Read the model definition and answer for the solid it produces. Units are mm, in the model's axes. Coordinates: 2 decimals unless noted, no trailing zeros. One line per item, written item: value. Start each with the question number.
1. Consider probe 1 along X at (y, z) = (-122.5, 5.25); probe 2 along X at (y, z) = (-123, 6.75); probe 3 along Z at (x, y) = (64.5, -119.5). Determine where each line is inside the solid, lowest interval first.
2. Determine the mould class of faces 1 (the face through (-4, -105, 3.463)), 2 (the face through (-4, -98, 16)), 3 (the face through (-1.85, -108.142, 8.112)) for opening direction Y: +Y half, -Y half, draft (parallel to the pull), parting line (faces both ways), or undercut.
3. Flat-ended cylindrical pins translate along their axes: pin 1 (2 mm diameter, centred on x = -36.5, z = 5.5, fed in from -Y); pin 2 (3 mm diameter, centred on x = -8, z = 5, fed in from -Y). Find the tip coordinate at first contact, or state that the pin passes through.
```python
from build123d import *

# Parameters (mm, degrees)
SKETCH1_W           = 169.5
SKETCH1_H           = 47.45
BOSS_EXTRUDE1_DEPTH = 32
SKETCH7_R           = 154
CUT_EXTRUDE5_DEPTH  = 32
SKETCH14_W          = 169.5
SKETCH14_H          = 16
BOSS_EXTRUDE2_DEPTH = 10


with BuildPart() as part:
    # Sketch1 → Boss-Extrude1 (new body)
    with BuildSketch(Plane.XY):
        with Locations((-3.10671108, -121.862113139)):
            Rectangle(SKETCH1_W, SKETCH1_H)
    extrude(amount=BOSS_EXTRUDE1_DEPTH)

    # Sketch7 → Cut-Extrude5 (cut)
    with BuildSketch(Plane.XY.offset(32)):
        with Locations((-3.10671108, -262.137113139)):
            Circle(SKETCH7_R)
    extrude(amount=-CUT_EXTRUDE5_DEPTH, mode=Mode.SUBTRACT)

    # Split2
    split(bisect_by=Plane(origin=(0, 0, 16), x_dir=(-1, 0, 0), z_dir=(0, 0, -1)), keep=Keep.TOP)

    # Cut-Sweep4: read off the stored shape, not the designer's step
    # Cut-Sweep4: loft between two sections, ruled curve by curve
    cut_sweep4_from = [
        Edge.make_bspline([(82.739791111, -124.333714197, 3.462903079), (82.375516408, -124.117363235, 3.462903079), (82.0018328, -123.896841508, 3.462903079), (68.621301032, -116.090106709, 3.462903079), (54.256669748, -110.065617594, 3.462903079), (24.029677947, -102.175579118, 3.462903079), (8.210854863, -100.312946687, 3.462903079), (-23.222204489, -101.051424681, 3.462903079), (-38.798228939, -103.637289837, 3.462903079), (-60.809960607, -110.444286671, 3.462903079), (-67.919122803, -113.18910099, 3.462903079), (-81.548905499, -119.521573676, 3.462903079), (-88.057522246, -123.118344791, 3.46290308), (-94.217927223, -127.000728785, 3.462903079)], [0, 0, 0, 0, 0.006836374, 0.006836374, 0.255127281, 0.255127281, 0.503418187, 0.503418187, 0.751709094, 0.751709094, 0.875854547, 0.875854547, 1, 1, 1, 1], 3),
        Edge.make_bspline([(82.696209972, -130.333555919, 3.462903079), (82.346471994, -130.117236359, 3.462903079), (81.986625524, -129.896841507, 3.462903079), (69.173615468, -122.090106764, 3.46290308), (55.332198525, -115.995213643, 3.462903079), (26.189346767, -107.801652521, 3.462903079), (10.873507842, -105.719561423, 3.462903079), (-19.594281231, -105.863843686, 3.462903079), (-34.749935159, -108.099853973, 3.462903079), (-56.203233344, -114.298356521, 3.462903079), (-63.148715446, -116.838422053, 3.462903079), (-76.467195094, -122.723221567, 3.462903079), (-82.839914651, -126.093721608, 3.462903079), (-88.893908679, -129.767464505, 3.462903079)], [0, 0, 0, 0, 0.006836374, 0.006836374, 0.255127281, 0.255127281, 0.503418187, 0.503418187, 0.751709094, 0.751709094, 0.875854547, 0.875854547, 1, 1, 1, 1], 3),
        Edge.make_line((-88.893908679, -129.767464505, 3.462903079), (-94.217927223, -127.000728785, 3.462903079)),
        Edge.make_line((82.696209972, -130.333555919, 3.462903079), (82.739791111, -124.333714197, 3.462903079)),
    ]
    cut_sweep4_to = [
        Edge.make_bspline([(82.739791111, -124.333714197, 16.002903079), (82.375516408, -124.117363235, 16.002903079), (82.0018328, -123.896841508, 16.002903079), (68.621301031, -116.090106708, 16.002903079), (54.256669748, -110.065617594, 16.002903079), (24.029677947, -102.175579118, 16.002903079), (8.210854863, -100.312946687, 16.002903079), (-23.222204489, -101.051424681, 16.002903079), (-38.798228939, -103.637289837, 16.00290308), (-60.809960607, -110.444286671, 16.002903079), (-67.919122803, -113.18910099, 16.002903079), (-81.548905499, -119.521573676, 16.002903079), (-88.057522246, -123.118344791, 16.002903079), (-94.217927223, -127.000728785, 16.002903079)], [0, 0, 0, 0, 0.006836374, 0.006836374, 0.255127281, 0.255127281, 0.503418187, 0.503418187, 0.751709094, 0.751709094, 0.875854547, 0.875854547, 1, 1, 1, 1], 3),
        Edge.make_bspline([(82.696209972, -130.333555919, 16.002903079), (82.346471994, -130.117236359, 16.002903079), (81.986625524, -129.896841507, 16.002903079), (69.173615467, -122.090106763, 16.00290308), (55.332198525, -115.995213643, 16.002903079), (26.189346767, -107.801652521, 16.002903079), (10.873507842, -105.719561423, 16.002903079), (-19.594281231, -105.863843686, 16.002903079), (-34.749935159, -108.099853973, 16.00290308), (-56.203233344, -114.298356521, 16.002903079), (-63.148715446, -116.838422053, 16.002903079), (-76.467195094, -122.723221567, 16.002903079), (-82.839914651, -126.093721608, 16.002903079), (-88.893908679, -129.767464505, 16.002903079)], [0, 0, 0, 0, 0.006836374, 0.006836374, 0.255127281, 0.255127281, 0.503418187, 0.503418187, 0.751709094, 0.751709094, 0.875854547, 0.875854547, 1, 1, 1, 1], 3),
        Edge.make_line((-88.893908679, -129.767464505, 16.002903079), (-94.217927223, -127.000728785, 16.002903079)),
        Edge.make_line((82.696209972, -130.333555919, 16.002903079), (82.739791111, -124.333714197, 16.002903079)),
    ]
    cut_sweep4 = Solid(Shell([*[Face.make_surface_from_curves(cut_sweep4_from[k], cut_sweep4_to[k]) for k in range(4)], Face(Wire(cut_sweep4_from)), Face(Wire(cut_sweep4_to))]))
    add(cut_sweep4, mode=Mode.SUBTRACT)

    # Sketch14 → Boss-Extrude2 (add)
    with BuildSketch(Plane(origin=(0, -98.137113139, 0), x_dir=(1, 0, 0), z_dir=(0, 1, 0))):
        with Locations((-3.10671108, -8)):
            Rectangle(SKETCH14_W, SKETCH14_H)
    extrude(amount=BOSS_EXTRUDE2_DEPTH)


solid = part.part
```
Answer block:
1. probe 1: x = -87.86 to -86.68, -75.64 to -68.05, 61.84 to 68.52, 79.57 to 81.64
1. probe 2: x = -87.86 to -87.56, -76.65 to -69.11, 62.9 to 69.53, 80.45 to 81.64
1. probe 3: z = 0 to 3.46
2. face 1: undercut
2. face 2: draft
2. face 3: -Y half
3. pin 1: stops at y = -112.03
3. pin 2: stops at y = -108.27
